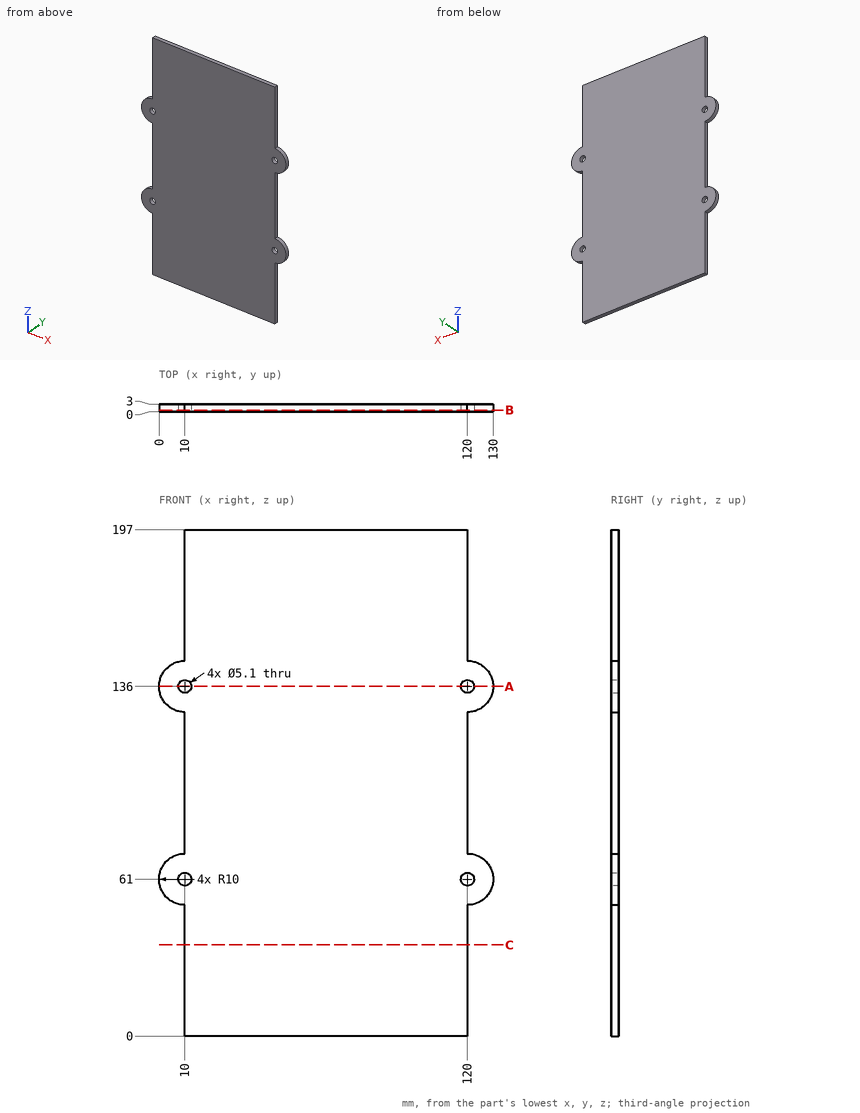
Part print with two shaded views. Sizes in mm from the minimum x, y, z corner. Round coordinates to 2 decimals unless told otherwise and drop trailing zeros. Loops run counter-clockwise (first coordinate to the right, second up) from the corner with the lowest first, then second, coordinate; pieces in that order, holes last. Notation, with made-up numbers: M 1,-38.75 L 41,-38.75 A9 ccw 41,-27.75 Z; hole C 46.5,-3 d4. An arc over 180 degrees is marked long. Return JSON: item names as keys, results as strings. Group by question number.
(1) Saw through at A-A, the plane z = 136. List the corners of the cut face in (x, y), and give its area (3 significant figures).
(2) Saw through at B-B, the plane y = 0.65. List the corners of the cut face in (x, z), and give its area (3 significant figures).
(3) Drop a flat-ended pin along its axis: P1, Ø1.5, axis at y = 2, z = 52.5, coming from the -X side. Give the stop position or say it passes through.
(4) Wall check: probe 1 along X at (y, z) = (0.9, 136); probe 2 along X at (y, z) = (1.25, 15.5); probe 3 along Z at (x, y) = (6.5, 2). Give the ranges that are in metal, low to high. Write a range as [from, to].
(5) Saw through at C-C, the plane z = 35.5. List the corners of the cut face in (x, y), and give its area (3 significant figures).
Answer list:
{
 "1": {"outline": "M 0,0 L 7.45,0 L 7.45,3 L 0,3 Z; M 12.55,0 L 117.45,0 L 117.45,3 L 12.55,3 Z; M 122.55,0 L 130,0 L 130,3 L 122.55,3 Z", "area": "359 mm2"},
 "2": {"outline": "M 10,0 L 120,0 L 120,51 A10 ccw 120,71 L 120,126 A10 ccw 120,146 L 120,197 L 10,197 L 10,146 A10 ccw 10,126 L 10,71 A10 ccw 10,51 Z; hole C 10,61 d5.1; hole C 10,136 d5.1; hole C 120,61 d5.1; hole C 120,136 d5.1", "area": "22,200 mm2"},
 "3": {"P1": "x = 3.68"},
 "4": {"probe 1": "[0, 7.45], [12.55, 117.45], [122.55, 130]", "probe 2": "[10, 120]", "probe 3": "[51.63, 70.37], [126.63, 145.37]"},
 "5": {"outline": "M 10,0 L 120,0 L 120,3 L 10,3 Z", "area": "330 mm2"}
}
